Part model, mm, in its own coordinate system. A direction names the side the tool comes from. Give positions to 0.01 mm unless a question says otherwise; leave off trailing zeros. Order: outer loops, then holes, each group sorted by start corner. A loop starts at its lowest first (then second) coordinate and runs counter-clockwise, first axis right, second up. Notation, with made-up numbers: M 1,20 L 37,20 A20 cw 37,31 Z; hole C 70,-11.75 d3. An arc over 180 degrees is marked long. One line per question, with ' | ' between items.
```python
from build123d import *

# Parameters (mm, degrees)
F0_W     = 35.116635263
F0_H     = 34.8606705666
F1_DEPTH = 800
F2_DEPTH = 600
F3_DEPTH = 370
F4_T     = -18
F5_DEPTH = 6


with BuildPart() as f1:
    # F0 (on Top) → F1 (new body)
    with BuildSketch(Plane.XY):
        with Locations((-17.5583176315, -17.4303352833)):
            Rectangle(F0_W, F0_H)
    extrude(amount=F1_DEPTH)

    # F2 (add): a face of the model
    f2_faces = [f1.faces().sort_by_distance(p)[0] for p in [
        (-17.5583176315, 0, 400),
    ]]
    extrude(f2_faces, amount=-F2_DEPTH)

    # F3 (add): a face of the model
    f3_faces = [f1.faces().sort_by_distance(p)[0] for p in [
        (0, -300, 400),
    ]]
    extrude(f3_faces, amount=-F3_DEPTH)

    # F4
    f4_openings = [f1.faces().sort_by_distance(p)[0] for p in [
        (-370, -300, 400),
    ]]
    offset(amount=F4_T, openings=f4_openings)

    # F5 (add): a face of the model
    f5_faces = [f1.faces().sort_by_distance(p)[0] for p in [
        (0, -300, 400),
    ]]
    extrude(f5_faces, amount=F5_DEPTH)


solid = f1.part
```
1. Probe L1, parallel to Z at x = -287, y = -364; L2, parallel to Y at x = -274.5, z = 473; L3, parallel to X at y = -328.5, z = 204.5. List the from-to ranges inside material, lowest first. Write a range as from..to.
Worked out:
L1: z = 0..18, 782..800 | L2: y = -600..-582, -18..0 | L3: x = -18..6
2. Slice it at C-C on y = -478.5. Give the cut face in (x, z).
Worked out:
outline: M -370,0 L 6,0 L 6,800 L -370,800 L -370,782 L -18,782 L -18,18 L -370,18 Z
3. Tool access for faces 1 (the flat face through (-192, -582, 395)), 2 (the flat face through (-185, -304, 800)): list every direction of +Z, -Z, +X, -X, +Y, -Y with a clear straight run to the whole face (end or side of a thin tool).
Worked out:
face 1: -X | face 2: +Z, +X, -X, +Y, -Y
4. Drop a flat-ended pin along its axis: pin 1 (2 mm diameter, centred on y = -303, z = 148.5, fed in from -X). Give the stop position or say it passes through.
Worked out:
pin 1: stops at x = -18
5. Mould opens along Z. For faces 3 (the flat face through (-192, -296, 18)), 4 (the flat face through (-185, -296, 0)), 5 (the flat face through (6, -296, 394)) say: released by +Z, released by -Z, zero draft, split by the parting line, or undercut.
Worked out:
face 3: undercut | face 4: released by -Z | face 5: zero draft
6. Slice it at B-B on z = 626.5. Give the cut face in (x, y), then the cut area to 3 significant figures.
Worked out:
outline: M -370,-600 L 6,-600 L 6,0 L -370,0 L -370,-18 L -18,-18 L -18,-582 L -370,-582 Z | area: 27,100 mm2
7. Slice it at A-A on x = -327. Give the cut face in (y, z), then the cut area to 3 significant figures.
Worked out:
outline: M -600,0 L 0,0 L 0,800 L -600,800 Z; hole M -582,18 L -18,18 L -18,782 L -582,782 Z | area: 49,100 mm2
